from build123d import *

# Parameters (mm, degrees)
SKETCH1_R           = 58
BOSS_EXTRUDE1_DEPTH = 4
SKETCH2_W           = 4
SKETCH2_H           = 54
CUT_EXTRUDE1_DEPTH  = 83.121860671
CUT_EXTRUDE2_DEPTH  = 4


with BuildPart() as part:
    # Sketch1 → Boss-Extrude1 (new body)
    with BuildSketch(Plane(origin=(0, 0, 0), x_dir=(1, 0, 0), z_dir=(0, 1, 0))):
        with Locations(Location((0, 0, 0), (0, 0, 270))):
            Circle(SKETCH1_R)
    extrude(amount=BOSS_EXTRUDE1_DEPTH)

    # Sketch2 → Cut-Extrude1 (cut, through all)
    with BuildSketch(Plane(origin=(0, 4, 0), x_dir=(1, 0, 0), z_dir=(0, 1, 0))):
        with Locations((37, 0)):
            Rectangle(SKETCH2_W, SKETCH2_H)
        with Locations((-37, 0)):
            Rectangle(SKETCH2_W, SKETCH2_H)
    extrude(amount=-CUT_EXTRUDE1_DEPTH, mode=Mode.SUBTRACT)

    # Sketch3 → Cut-Extrude2 (cut)
    with BuildSketch(Plane(origin=(0, 4, 0), x_dir=(1, 0, 0), z_dir=(0, 1, 0))):
        with BuildLine():
            Line((-15, 6), (15, 6))
            ThreePointArc((15, 6), (17, 8), (15, 10))
            Line((15, 10), (-15, 10))
            ThreePointArc((-15, 10), (-17, 8), (-15, 6))
        make_face()
        with BuildLine():
            Line((-15, 14), (15, 14))
            ThreePointArc((15, 14), (17, 16), (15, 18))
            Line((15, 18), (-15, 18))
            ThreePointArc((-15, 18), (-17, 16), (-15, 14))
        make_face()
        with BuildLine():
            Line((-15, -10), (15, -10))
            ThreePointArc((15, -10), (17, -8), (15, -6))
            Line((15, -6), (-15, -6))
            ThreePointArc((-15, -6), (-17, -8), (-15, -10))
        make_face()
        with BuildLine():
            Line((-15, -26), (15, -26))
            ThreePointArc((15, -26), (17, -24), (15, -22))
            Line((15, -22), (-15, -22))
            ThreePointArc((-15, -22), (-17, -24), (-15, -26))
        make_face()
        with BuildLine():
            Line((-15, 2), (15, 2))
            ThreePointArc((15, 2), (17, 0), (15, -2))
            Line((15, -2), (-15, -2))
            ThreePointArc((-15, -2), (-17, 0), (-15, 2))
        make_face()
        with BuildLine():
            Line((-15, 26), (15, 26))
            ThreePointArc((15, 26), (17, 24), (15, 22))
            Line((15, 22), (-15, 22))
            ThreePointArc((-15, 22), (-17, 24), (-15, 26))
        make_face()
        with BuildLine():
            Line((-15, -14), (15, -14))
            ThreePointArc((15, -14), (17, -16), (15, -18))
            Line((15, -18), (-15, -18))
            ThreePointArc((-15, -18), (-17, -16), (-15, -14))
        make_face()
    extrude(amount=-CUT_EXTRUDE2_DEPTH, mode=Mode.SUBTRACT)


solid = part.part
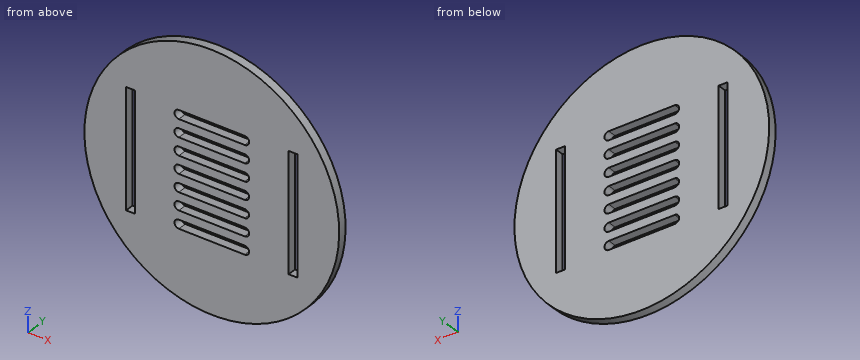
Work out the finished part from the listing and answer in its coordinate system (mm). Give positions to 0.01 mm unless a question says otherwise; leave off trailing zeros. Loops run counter-clockwise (first coordinate to the right, second up) from the corner with the lowest first, then second, coordinate; pieces in that order, holes last. Notation, with made-up numbers: (68.25, 45) - (74.25, 45) arc R17 cw to (74.25, 63) - close; hole circle Ø3 at (34.5, -35.75). An arc over 180 degrees is marked (long way). Answer in a Markdown table with one row per item. Add a question column.
Q1. The part is cut by section A-A (x = 0). State how many separate pieces and enclosed holes the cut face has, and give its area (3 significant figures).
Q2. The part is cut by section B-B (z = 3.5). Determine the outline of the cut face in (x, y).
Q3. Each of these flat-tipped pins is pushed along its axis until it touches: P1, Ø1.2, axis at x = 7, y = 3, coming from the -Z side; P2, Ø1.5, axis at x = 36, z = 12, coming from the -Y side; P3, Ø1.2, axis at y = 1.5, z = 1.5, coming from the -X side; P4, Ø2, axis at x = 3.5, y = 3, coming from the +Z side. Where does it stop, or does it pass through?
Q4. The part is cut by section C-C (z = 16). Determine the outline of the cut face in (x, y), and give its area (3 significant figures).
Q5. Consider line 1 along X through (y, z) = (1.35, 0); line 2 along X through (y, z) = (0.3, 6.5); line 3 along X through (y, z) = (2.25, -5). Determine where each line is inside the solid, lowest interval first.
Solution:
| question | item | result |
|---|---|---|
| 1 | separate pieces | 8 |
| 1 | enclosed holes | 0 |
| 1 | area | 352 mm² |
| 2 | outline | (-57.89, 0) - (-39, 0) - (-39, 4) - (-57.89, 4) - close; (-35, 0) - (35, 0) - (35, 4) - (-35, 4) - close; (39, 0) - (57.89, 0) - (57.89, 4) - (39, 4) - close |
| 3 | P1 | stops at z = -57.65 |
| 3 | P2 | passes through |
| 3 | P3 | stops at x = -57.99 |
| 3 | P4 | stops at z = 57.95 |
| 4 | outline | (-55.75, 0) - (-39, 0) - (-39, 4) - (-55.75, 4) - close; (-35, 0) - (-17, 0) - (-17, 4) - (-35, 4) - close; (17, 0) - (35, 0) - (35, 4) - (17, 4) - close; (39, 0) - (55.75, 0) - (55.75, 4) - (39, 4) - close |
| 4 | area | 278 mm² |
| 5 | line 1 | x = -58 to -39, -35 to -17, 17 to 35, 39 to 58 |
| 5 | line 2 | x = -57.63 to -39, -35 to -16.32, 16.32 to 35, 39 to 57.63 |
| 5 | line 3 | x = -57.78 to -39, -35 to 35, 39 to 57.78 |
